```python
from build123d import *

# Parameters (mm, degrees)
BOSS_EXTRUDE1_DEPTH  = 3.5
BOSS_EXTRUDE2_DEPTH  = 21
SKETCH3_W            = 23
SKETCH3_H            = 39
BOSS_EXTRUDE3_DEPTH  = 2.5
SKETCH5_W            = 21.5
SKETCH5_H            = 25
SKETCH5_W_2          = 7.07
SKETCH5_H_2          = 19.04
BOSS_EXTRUDE5_DEPTH  = 2.5
SKETCH6_W            = 7.07
SKETCH6_H            = 5.9
BOSS_EXTRUDE6_DEPTH  = 20
BOSS_EXTRUDE7_DEPTH  = 23
FILLET1_SIZE         = 10
SKETCH9_R            = 2.475
BOSS_EXTRUDE8_DEPTH  = 9
FILLET2_R            = 0.5
SKETCH10_R           = 1.65
CUT_EXTRUDE1_DEPTH   = 9
SKETCH11_W           = 0.2
SKETCH11_H           = 20
CUT_EXTRUDE2_DEPTH   = 9
CUT_EXTRUDE3_DEPTH   = 9
FILLET3_SIZE         = 3
BOSS_EXTRUDE9_DEPTH  = 5
SKETCH14_R           = 1.747814763
SKETCH14_R_2         = 1.6
CUT_EXTRUDE4_DEPTH   = 15
BOSS_EXTRUDE10_DEPTH = 35
SKETCH17_W           = 110
SKETCH17_H           = 3.5
BOSS_EXTRUDE11_DEPTH = 15
SKETCH18_W           = 161.485932181
SKETCH18_H           = 44
CUT_EXTRUDE5_DEPTH   = 63
SKETCH19_W           = 4.328620931
SKETCH19_H           = 15
BOSS_EXTRUDE12_DEPTH = 35
FILLET4_SIZE         = 1
SKETCH20_W           = 4.640065176
SKETCH20_H           = 12
SKETCH20_R           = 1.55
SKETCH20_W_2         = 10
SKETCH20_H_2         = 5
BOSS_EXTRUDE13_DEPTH = 4
SKETCH21_W           = 32
SKETCH21_H           = 15.5
CUT_EXTRUDE6_DEPTH   = 14
FILLET5_SIZE         = 1
FILLET6_SIZE         = 4


with BuildPart() as part:
    # Sketch1 → Boss-Extrude1 (new body)
    with BuildSketch(Plane(origin=(0, 0, 0), x_dir=(1, 0, 0), z_dir=(0, 1, 0))):
        Polygon((0, 40), (23, 40), (23, 79), (0, 79), (0, 100), (110, 100), (110, 79), (87, 79), (87, 40), (110, 40), (110, 20), (80, 0), (30, 0), (0, 20), align=None)
    extrude(amount=BOSS_EXTRUDE1_DEPTH)

    # Sketch2 → Boss-Extrude2 (add)
    with BuildSketch(Plane(origin=(0, 3.5, 0), x_dir=(1, 0, 0), z_dir=(0, 1, 0))):
        Polygon((0, 79), (23, 79), (23, 40), (0, 40), (0, 37.5), (25.5, 37.5), (25.5, 81.5), (0, 81.5), align=None)
        Polygon((110, 81.5), (84.5, 81.5), (84.5, 37.5), (110, 37.5), (110, 40), (87, 40), (87, 79), (110, 79), align=None)
    extrude(amount=BOSS_EXTRUDE2_DEPTH)

    # Sketch3 → Boss-Extrude3 (add)
    with BuildSketch(Plane(origin=(0, 24.5, 0), x_dir=(1, 0, 0), z_dir=(0, 1, 0))):
        with Locations((11.5, 59.5)):
            Rectangle(SKETCH3_W, SKETCH3_H)
        with Locations((98.5, 59.5)):
            Rectangle(SKETCH3_W, SKETCH3_H)
    extrude(amount=-BOSS_EXTRUDE3_DEPTH)

    # Sketch5 → Boss-Extrude5 (add)
    with BuildSketch(Plane(origin=(0, 24.5, 0), x_dir=(1, 0, 0), z_dir=(0, 1, 0))):
        with Locations((120.75, 50)):
            Rectangle(SKETCH5_W, SKETCH5_H)
        with Locations((-10.75, 50)):
            Rectangle(SKETCH5_W, SKETCH5_H)
        with Locations((29.035, 47.02)):
            Rectangle(SKETCH5_W_2, SKETCH5_H_2)
        with Locations((80.965, 47.02)):
            Rectangle(SKETCH5_W_2, SKETCH5_H_2)
    extrude(amount=-BOSS_EXTRUDE5_DEPTH)

    # Sketch6 → Boss-Extrude6 (add)
    with BuildSketch(Plane(origin=(0, 24.5, 0), x_dir=(1, 0, 0), z_dir=(0, 1, 0))):
        with Locations((29.035, 53.59)):
            Rectangle(SKETCH6_W, SKETCH6_H)
        with Locations((80.965, 53.59)):
            Rectangle(SKETCH6_W, SKETCH6_H)
        with Locations((-17.965, 53.59)):
            Rectangle(SKETCH6_W, SKETCH6_H)
        with Locations((127.965, 53.59)):
            Rectangle(SKETCH6_W, SKETCH6_H)
    extrude(amount=BOSS_EXTRUDE6_DEPTH)

    # Sketch7 → Boss-Extrude7 (add)
    with BuildSketch(Plane(origin=(0, 24.5, 0), x_dir=(1, 0, 0), z_dir=(0, 1, 0))):
        Polygon((0, 81.5), (25.5, 81.5), (25.5, 79), (0, 79), (-21.5, 79), (-21.5, 81.5), align=None)
        Polygon((110, 79), (84.5, 79), (84.5, 81.5), (110, 81.5), (131.5, 81.5), (131.5, 79), align=None)
    extrude(amount=BOSS_EXTRUDE7_DEPTH)

    # Fillet1
    # the kernel refuses this chamfer: 10 mm, written as the material it adds along each edge
    with BuildSketch(Plane(origin=(0, 22, -40), x_dir=(0.027495876610586372, -0.9996219169112968, 0), z_dir=(0, 0, 1)), Plane(origin=(110, 22, -37.5), x_dir=(-0.027495876610586317, -0.9996219169112968, 0), z_dir=(0, 0, -1)), Plane(origin=(110, 24.5, -81.5), x_dir=(0.9996219169112968, 0.027495876610586317, 0), z_dir=(0, 0, 1))) as fillet1_piece_1:
        Polygon((FILLET1_SIZE * 0.999621916911, -FILLET1_SIZE * 0.0274958766106), (-FILLET1_SIZE * 0.0274958766106, -FILLET1_SIZE * 0.999621916911), (0, 0), align=None)
    extrude(amount=2.5)
    with BuildSketch(Plane(origin=(0, 24.5, -79), x_dir=(0.027495876610586372, -0.9996219169112968, 0), z_dir=(0, 0, -1))) as fillet1_piece_2:
        Polygon((FILLET1_SIZE * 0.999621916911, FILLET1_SIZE * 0.0274958766106), (-FILLET1_SIZE * 0.0274958766106, FILLET1_SIZE * 0.999621916911), (0, 0), align=None)
    extrude(amount=2.5)

    # Sketch9 → Boss-Extrude8 (add)
    with BuildSketch(Plane(origin=(0, 0, -81.5), x_dir=(-1, 0, 0), z_dir=(0, 0, -1))):
        with Locations(Location((-114.55, 34.35, 0), (0, 0, 180))):
            Circle(SKETCH9_R)
        with Locations(Location((4.55, 34.35, 0), (0, 0, 180))):
            Circle(SKETCH9_R)
    extrude(amount=BOSS_EXTRUDE8_DEPTH)

    # Fillet2
    fillet2_edges = [part.edges().sort_by_distance(p)[0] for p in [
        (112.075, 34.35, -90.5),
        (-7.025, 34.35, -90.5),
    ]]
    fillet(fillet2_edges, radius=FILLET2_R)

    # Sketch10 → Cut-Extrude1 (cut)
    with BuildSketch(Plane.XY.offset(-50.64)):
        with Locations((129.16, 39.27)):
            Circle(SKETCH10_R)
        with Locations((129.16, 29.43)):
            Circle(SKETCH10_R)
        with Locations((79.77, 39.27)):
            Circle(SKETCH10_R)
        with Locations((79.77, 29.43)):
            Circle(SKETCH10_R)
        with Locations((-19.16, 29.43)):
            Circle(SKETCH10_R)
        with Locations((-19.16, 39.27)):
            Circle(SKETCH10_R)
        with Locations(Location((30.23, 39.27, 0), (0, 0, 180))):
            Circle(SKETCH10_R)
        with Locations(Location((30.23, 29.43, 0), (0, 0, 180))):
            Circle(SKETCH10_R)
    extrude(amount=-CUT_EXTRUDE1_DEPTH, mode=Mode.SUBTRACT)

    # Sketch11 → Cut-Extrude2 (cut)
    with BuildSketch(Plane.XY.offset(-50.64)):
        with Locations((-14.53, 34.5)):
            Rectangle(SKETCH11_W, SKETCH11_H)
        with Locations((25.6, 34.5)):
            Rectangle(SKETCH11_W, SKETCH11_H)
        with Locations((84.4, 34.5)):
            Rectangle(SKETCH11_W, SKETCH11_H)
        with Locations((124.53, 34.5)):
            Rectangle(SKETCH11_W, SKETCH11_H)
    extrude(amount=-CUT_EXTRUDE2_DEPTH, mode=Mode.SUBTRACT)

    # Sketch12 → Cut-Extrude3 (cut)
    with BuildSketch(Plane(origin=(0, 0, -81.5), x_dir=(-1, 0, 0), z_dir=(0, 0, -1))):
        Polygon((-108, 47.5), (-84.5, 25.5), (-84.5, 47.5), align=None)
        Polygon((-25.5, 25.5), (-25.5, 47.5), (-2, 47.5), align=None)
        Polygon((-120, 24.5), (-131.5, 36), (-131.5, 24.5), align=None)
        Polygon((10, 24.5), (21.5, 36), (21.5, 24.5), align=None)
    extrude(amount=-CUT_EXTRUDE3_DEPTH, mode=Mode.SUBTRACT)

    # Fillet3
    fillet3_edges = [part.edges().sort_by_distance(p)[0] for p in [
        (0, 23.25, -62.5),
        (110, 23.25, -62.5),
    ]]
    chamfer(fillet3_edges, length=FILLET3_SIZE)

    # Sketch13 → Boss-Extrude9 (add)
    with BuildSketch(Plane(origin=(0, 3.5, 0), x_dir=(1, 0, 0), z_dir=(0, 1, 0))):
        Polygon((0, 30.5), (32.5, 30.5), (32.5, 88.5), (0, 88.5), (0, 81.5), (25.5, 81.5), (25.5, 37.5), (0, 37.5), align=None)
        Polygon((84.5, 37.5), (110, 37.5), (110, 30.5), (77.5, 30.5), (77.5, 88.5), (110, 88.5), (110, 81.5), (84.5, 81.5), align=None)
    extrude(amount=BOSS_EXTRUDE9_DEPTH)

    # Sketch14 → Cut-Extrude4 (cut)
    with BuildSketch(Plane(origin=(0, 8.5, 0), x_dir=(1, 0, 0), z_dir=(0, 1, 0))):
        with Locations(Location((7.25, 34, 0), (0, 0, 270))):
            Circle(SKETCH14_R)
        with Locations(Location((7.25, 85, 0), (0, 0, 270))):
            Circle(SKETCH14_R_2)
        with Locations(Location((29, 34, 0), (0, 0, 270))):
            Circle(SKETCH14_R_2)
        with Locations(Location((29, 59.5, 0), (0, 0, 270))):
            Circle(SKETCH14_R_2)
        with Locations(Location((29, 85, 0), (0, 0, 270))):
            Circle(SKETCH14_R_2)
        with Locations(Location((81, 34, 0), (0, 0, 90))):
            Circle(SKETCH14_R_2)
        with Locations(Location((102.75, 34, 0), (0, 0, 90))):
            Circle(SKETCH14_R)
        with Locations(Location((81, 59.5, 0), (0, 0, 90))):
            Circle(SKETCH14_R_2)
        with Locations(Location((81, 85, 0), (0, 0, 90))):
            Circle(SKETCH14_R_2)
        with Locations(Location((102.75, 85, 0), (0, 0, 90))):
            Circle(SKETCH14_R_2)
    extrude(amount=-CUT_EXTRUDE4_DEPTH, mode=Mode.SUBTRACT)

    # Sketch15 → Boss-Extrude10 (add)
    with BuildSketch(Plane(origin=(0, 3.5, 0), x_dir=(1, 0, 0), z_dir=(0, 1, 0))):
        Polygon((110, 20), (80, 0), (30, 0), (0, 20), (6.309714732, 20), (31.059714732, 3.5), (78.940285268, 3.5), (103.405491726, 19.81009599), align=None)
    extrude(amount=BOSS_EXTRUDE10_DEPTH)

    # Sketch17 → Boss-Extrude11 (add)
    with BuildSketch(Plane(origin=(0, 0, -100), x_dir=(-1, 0, 0), z_dir=(0, 0, -1))):
        with Locations((-55, 1.75)):
            Rectangle(SKETCH17_W, SKETCH17_H)
    extrude(amount=BOSS_EXTRUDE11_DEPTH)

    # Sketch18 → Cut-Extrude5 (cut)
    with BuildSketch(Plane(origin=(0, 0, -88.5), x_dir=(-1, 0, 0), z_dir=(0, 0, -1))):
        with Locations((-59.242966091, 25.5)):
            Rectangle(SKETCH18_W, SKETCH18_H)
    extrude(amount=-CUT_EXTRUDE5_DEPTH, mode=Mode.SUBTRACT)


with BuildPart() as body_2:
    # of the pieces the cut leaves, the one that is kept (cut_extrude5_keep)
    add(part.part.solids().sort_by_distance((0, 3.5, -79))[0])

    # Sketch19 → Boss-Extrude12 (add)
    with BuildSketch(Plane(origin=(0, 3.5, 0), x_dir=(1, 0, 0), z_dir=(0, 1, 0))):
        with Locations((107.835689535, 107.5)):
            Rectangle(SKETCH19_W, SKETCH19_H)
        with Locations((2.164310466, 107.5)):
            Rectangle(SKETCH19_W, SKETCH19_H)
    extrude(amount=BOSS_EXTRUDE12_DEPTH)

    # Fillet4
    fillet4_edges = [body_2.edges().sort_by_distance(p)[0] for p in [
        (0, 21, -100),
        (4.328620931, 21, -100),
        (110, 21, -100),
        (105.671379069, 21, -100),
    ]]
    chamfer(fillet4_edges, length=FILLET4_SIZE)

    # Sketch20 → Boss-Extrude13 (add)
    # profile 1 of 6: a face of its own
    with BuildSketch(Plane(origin=(0, 0, -115), x_dir=(-1, 0, 0), z_dir=(0, 0, -1))):
        with Locations((-112.320032588, 32.5)):
            Rectangle(SKETCH20_W, SKETCH20_H)
        with Locations((-112.320032588, 32.5)):
            Circle(SKETCH20_R, mode=Mode.SUBTRACT)
    # profile 2 of 6: a face of its own
    with BuildSketch(Plane(origin=(0, 0, -115), x_dir=(-1, 0, 0), z_dir=(0, 0, -1))):
        with Locations((-112.320032588, 6)):
            Rectangle(SKETCH20_W, SKETCH20_H)
        with Locations((-112.320032588, 6)):
            Circle(SKETCH20_R, mode=Mode.SUBTRACT)
    # profile 3 of 6: a face of its own
    with BuildSketch(Plane(origin=(0, 0, -115), x_dir=(-1, 0, 0), z_dir=(0, 0, -1))):
        with Locations((2.320032588, 6)):
            Rectangle(SKETCH20_W, SKETCH20_H)
        with Locations(Location((2.320032588, 6, 0), (0, 0, 180))):
            Circle(SKETCH20_R, mode=Mode.SUBTRACT)
    # profile 4 of 6: a face of its own
    with BuildSketch(Plane(origin=(0, 0, -115), x_dir=(-1, 0, 0), z_dir=(0, 0, -1))):
        with Locations((2.320032588, 32.5)):
            Rectangle(SKETCH20_W, SKETCH20_H)
        with Locations(Location((2.320032588, 32.5, 0), (0, 0, 180))):
            Circle(SKETCH20_R, mode=Mode.SUBTRACT)
    # profile 5 of 6: a face of its own
    with BuildSketch(Plane(origin=(0, 0, -115), x_dir=(-1, 0, 0), z_dir=(0, 0, -1))):
        with Locations((-74.4, 6)):
            Rectangle(SKETCH20_W_2, SKETCH20_H_2)
        with Locations((-74.4, 6)):
            Circle(SKETCH20_R, mode=Mode.SUBTRACT)
    # profile 6 of 6: a face of its own
    with BuildSketch(Plane(origin=(0, 0, -115), x_dir=(-1, 0, 0), z_dir=(0, 0, -1))):
        with Locations((-35.6, 6)):
            Rectangle(SKETCH20_W_2, SKETCH20_H_2)
        with Locations(Location((-35.6, 6, 0), (0, 0, 180))):
            Circle(SKETCH20_R, mode=Mode.SUBTRACT)
    extrude(amount=-BOSS_EXTRUDE13_DEPTH)

    # Sketch21 → Cut-Extrude6 (cut)
    with BuildSketch(Plane.XY):
        with Locations((55, 20.75)):
            Rectangle(SKETCH21_W, SKETCH21_H)
    extrude(amount=-CUT_EXTRUDE6_DEPTH, mode=Mode.SUBTRACT)

    # Fillet5
    fillet5_edges = [body_2.edges().sort_by_distance(p)[0] for p in [
        (114.640065176, 26.5, -113),
        (114.640065176, 38.5, -113),
        (114.640065176, 0, -113),
        (114.640065176, 12, -113),
        (-4.640065176, 12, -113),
        (-4.640065176, 0, -113),
        (-4.640065176, 38.5, -113),
        (-4.640065176, 26.5, -113),
        (79.4, 8.5, -113),
        (69.4, 8.5, -113),
        (30.6, 8.5, -113),
        (40.6, 8.5, -113),
    ]]
    chamfer(fillet5_edges, length=FILLET5_SIZE)

    # Fillet6
    fillet6_edges = [body_2.edges().sort_by_distance(p)[0] for p in [
        (105.671379069, 3.5, -108),
        (4.328620931, 3.5, -108),
    ]]
    chamfer(fillet6_edges, length=FILLET6_SIZE)


solid = body_2.part
```
CAD build for the part. Positions are in the model's coordinates, mm. A direction names the side the tool comes from. Round coordinates to 2 decimals unless told otherwise and drop trailing zeros. Loops run counter-clockwise (first coordinate to the right, second up) from the corner with the lowest first, then second, coordinate; pieces in that order, holes last. Notation, with made-up numbers: M -33,13.5 L -7,13.5 A24 cw -7,31.5 Z; hole C 24,79.25 d6. An arc over 180 degrees is marked long. Return JSON: item names as keys, results as strings. Group by question number.
(1) Saw through at C-C, the plane z = -85. List the corners of the cut face in (x, y).
(2) Wall check: probe 1 along X at (y, z) = (2.2, -85); probe 2 along X at (y, z) = (2.85, -34); probe 3 along Y at (x, z) = (54, -51). Give the ranges that are in metal, low to high. Write a range as [from, to].
(3) Tool access for faces 1 (the flat face through (30.6, 5, -113)), 2 (the flat face through (39, 21, -2)), 3 (the flat face through (11, 2, -79)), 4 (the flat face through (76, 5, -111)), 5 (the flat face through (-2, 12, -113)): list every direction of +Z, -Z, +X, -X, +Y, -Y with a clear straight run to the whole face (end or side of a thin tool).
(4) Saw through at B-B, the plane y = 18. List the corners of the cut face in (x, z).
(5) Mould opens along Z. For faces 6 (the cylindrical face through (110.842, 32.966, -113.028)), 7 (the flat face through (-1.3, 7.4, -111)), 8 (the cylindrical face through (80.519, 1.774, -61.026)) say: +Z half, -Z half, draft (parallel to the pull), parting line (faces both ways), or undercut.
(6) Saw through at A-A, the plane x = 56. List the corners of the cut face in (y, z).
(7) Drop flat-ended pins along their axis: P1, Ø10, axis at x = 73.5, y = 14, coming from the -Z side; P2, Ø1, axis at y = 2.5, z = -26.5, coming from the +X side; P3, Ø2, axis at x = 96.5, y = 14.5, coming from the -Z side; P4, Ø5, axis at x = 78, y = 10.5, coming from the +Z side. Give the stop position or say it passes through.
(8) Saw through at D-D, the plane y = 36. List the corners of the cut face in (x, z), and give its area (3 significant figures).
Answer list:
{
 "1": {"outline": "M 0,0 L 5.65,0 L 5.65,3.5 L 0,3.5 Z; M 8.85,0 L 27.4,0 L 27.4,3.5 L 8.85,3.5 Z; M 30.6,0 L 79.4,0 L 79.4,3.5 L 30.6,3.5 Z; M 82.6,0 L 101.15,0 L 101.15,3.5 L 82.6,3.5 Z; M 104.35,0 L 110,0 L 110,3.5 L 104.35,3.5 Z"},
 "2": {"probe 1": "[0, 5.65], [8.85, 27.4], [30.6, 79.4], [82.6, 101.15], [104.35, 110]", "probe 2": "[0, 5.5], [9, 27.4], [30.6, 79.4], [82.6, 101], [104.5, 110]", "probe 3": "[0, 3.5]"},
 "3": {"face 1": "-Z, +Y", "face 2": "+Z, -Z", "face 3": "-X, +Y, -Y", "face 4": "+Y", "face 5": "+Z, -Z, -X"},
 "4": {"outline": "M 0,-115 L 4.33,-115 L 4.33,-101 L 3.33,-100 L 1,-100 L 0,-101 Z; M 0,-20 L 6.31,-20 L 31.06,-3.5 L 39,-3.5 L 39,0 L 30,0 Z; M 71,-3.5 L 78.94,-3.5 L 103.41,-19.81 L 110,-20 L 80,0 L 71,0 Z; M 105.67,-115 L 110,-115 L 110,-101 L 109,-100 L 106.67,-100 L 105.67,-101 Z"},
 "5": {"face 6": "draft", "face 7": "+Z half", "face 8": "undercut"},
 "6": {"outline": "M 0,-115 L 3.5,-115 L 3.5,-3.5 L 13,-3.5 L 13,0 L 0,0 Z; M 28.5,-3.5 L 38.5,-3.5 L 38.5,0 L 28.5,0 Z"},
 "7": {"P1": "z = -3.5", "P2": "x = 110", "P3": "z = -15.87", "P4": "z = 0"},
 "8": {"outline": "M -4.64,-115 L 4.33,-115 L 4.33,-101 L 3.33,-100 L 1,-100 L 0,-101 L 0,-111 L -4.64,-111 Z; M 0,-20 L 6.31,-20 L 31.06,-3.5 L 78.94,-3.5 L 103.41,-19.81 L 110,-20 L 80,0 L 30,0 Z; M 105.67,-115 L 114.64,-115 L 114.64,-111 L 110,-111 L 110,-101 L 109,-100 L 106.67,-100 L 105.67,-101 Z", "area": "566 mm2"}
}
